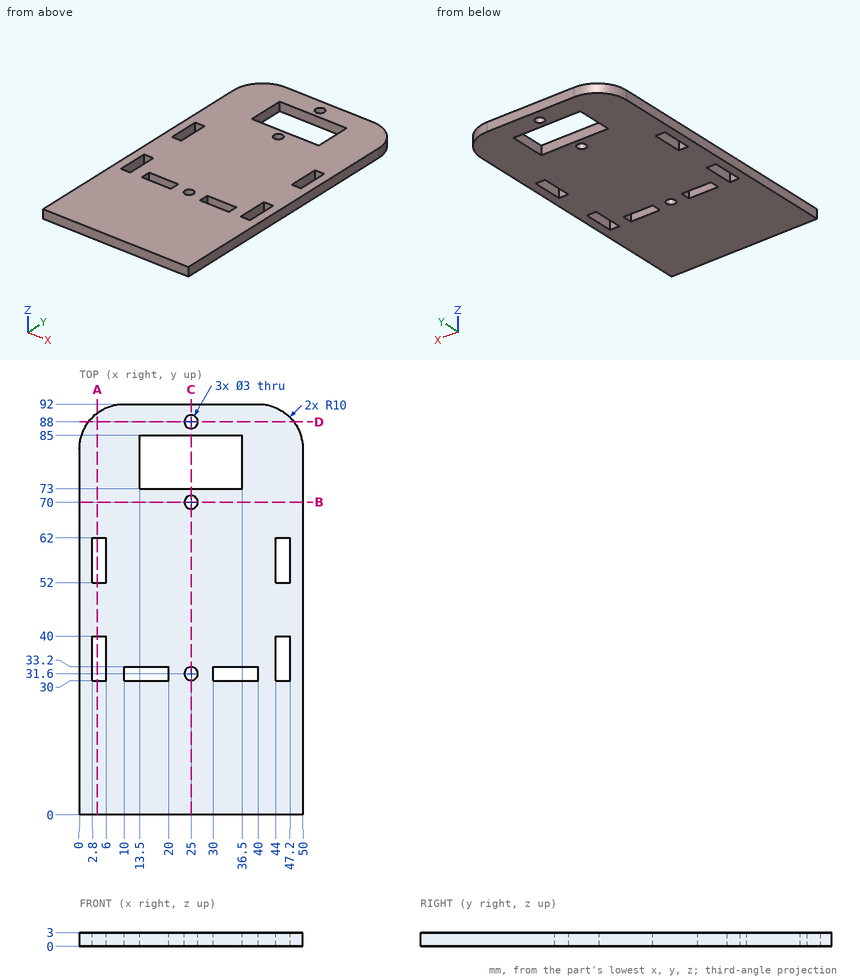
The figure shows three views and two pictorial views of one solid part (mm, origin at its lowest corner). Answer the questions. Coordinates: 2 decimals unless noted, no trailing zeros. Loops run counter-clockwise (first coordinate to the right, second up) from the corner with the lowest first, then second, coordinate; pieces in that order, holes last. Notation, with made-up numbers: (81, -18) -> (98, -18) arc R24 ccw to (98, 18) -> close; hole circle Ø11 at (75.5, 43.5). An arc over 180 degrees is marked (long way). Return JSON: item names as keys, results as strings. Group by question number.
(1) A cutting plane is placed at D-D on y = 88. Write down the section's boundary in (x, z), and give its area (3 significant figures).
(2) A cutting plane is placed at A-A on x = 4. Write down the section's boundary in (y, z), and give its area (3 significant figures).
(3) A cutting plane is placed at C-C on x = 25. Write down the section's boundary in (y, z).
(4) Find the intervals of material crossed by probe 1 along Y at (x, z) = (36, 0.3); probe 2 along Y at (x, z) = (25, 1.35); probe 3 along Y at (x, z) = (11, 0.3), in increasing order. Write a range as from..to.
(5) A cutting plane is placed at B-B on y = 70. Write down the section's boundary in (x, z), and give its area (3 significant figures).
(6) Given pin 1 Ø1.5 at (x, z) = (41, 2) entering from +Y; pin 2 Ø1.5 at (x, z) = (36, 2) entering from -Y, each flat-ended and moving along its own axis, determine where each tip first touches the part or whether it passes through.
The answers:
{
 "1": {"outline": "(2, 0) -> (23.5, 0) -> (23.5, 3) -> (2, 3) -> close; (26.5, 0) -> (48, 0) -> (48, 3) -> (26.5, 3) -> close", "area": "129 mm^2"},
 "2": {"outline": "(0, 0) -> (30, 0) -> (30, 3) -> (0, 3) -> close; (40, 0) -> (52, 0) -> (52, 3) -> (40, 3) -> close; (62, 0) -> (90, 0) -> (90, 3) -> (62, 3) -> close", "area": "210 mm^2"},
 "3": {"outline": "(0, 0) -> (30.1, 0) -> (30.1, 3) -> (0, 3) -> close; (33.1, 0) -> (68.5, 0) -> (68.5, 3) -> (33.1, 3) -> close; (71.5, 0) -> (73, 0) -> (73, 3) -> (71.5, 3) -> close; (85, 0) -> (86.5, 0) -> (86.5, 3) -> (85, 3) -> close; (89.5, 0) -> (92, 0) -> (92, 3) -> (89.5, 3) -> close"},
 "4": {"probe 1": "y = 0..30, 33.2..73, 85..92", "probe 2": "y = 0..30.1, 33.1..68.5, 71.5..73, 85..86.5, 89.5..92", "probe 3": "y = 0..30, 33.2..92"},
 "5": {"outline": "(0, 0) -> (23.5, 0) -> (23.5, 3) -> (0, 3) -> close; (26.5, 0) -> (50, 0) -> (50, 3) -> (26.5, 3) -> close", "area": "141 mm^2"},
 "6": {"pin 1": "stops at y = 92", "pin 2": "stops at y = 0"}
}
